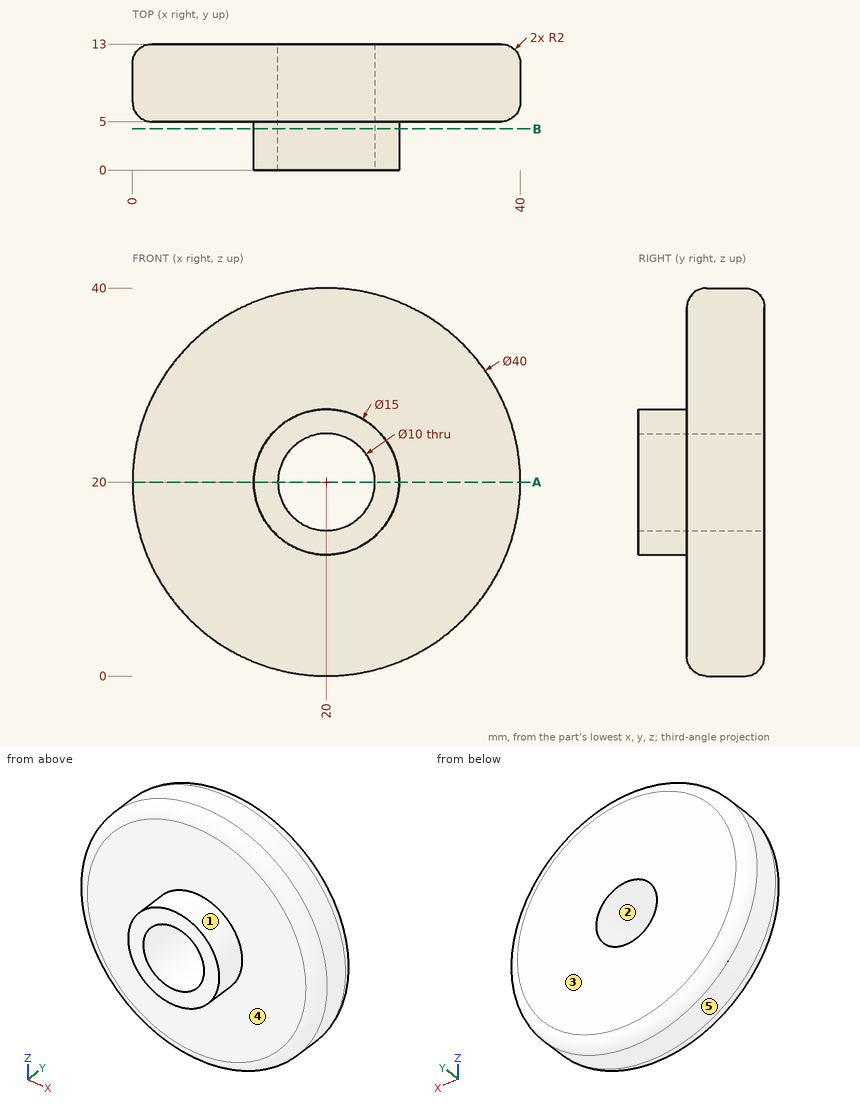
Study the drawing (mm; zero at the part's minimum x, y, z) and answer. A direction names the side the tool comes from. Give positions to 0.01 mm unless a question says otherwise; leave off trailing zeros. Loops run counter-clockwise (first coordinate to the right, second up) from the corner with the lowest first, then second, coordinate; pieces in that order, holes last. Notation, with made-up numbers: (22, 13.25) - (80, 13.25) arc R28 cw to (80, 35.25) - close; hole circle Ø11 at (4, 69.25). An arc over 180 degrees is marked (long way). One line per question, with ' | ' between items.
(1) The part is cut by section A-A (z = 20). Write down the section's boundary in (x, y).
Recorded:
outline: (0, 7) arc R2 ccw to (2, 5) - (12.5, 5) - (12.5, 0) - (15, 0) - (15, 13) - (2, 13) arc R2 ccw to (0, 11) - close; (25, 0) - (27.5, 0) - (27.5, 5) - (38, 5) arc R2 ccw to (40, 7) - (40, 11) arc R2 ccw to (38, 13) - (25, 13) - close
(2) Each of these flat-tipped pins is pushed along its axis until it touches: pin 1 Ø1 at (y, z) = (7.5, 16) entering from +X; pin 2 Ø5 at (y, z) = (9.5, 28) entering from -X; pin 3 Ø6 at (x, y) = (13.5, 8.5) entering from +Z; pin 4 Ø13 at (x, z) = (20, 20) entering from -Y. Where does it stop, or does it pass through?
Recorded:
pin 1: stops at x = 39.69 | pin 2: stops at x = 0.77 | pin 3: stops at z = 39.69 | pin 4: stops at y = 0
(3) The part is cut by section B-B (y = 4.25). Write down the section's boundary in (x, z).
Recorded:
outline: circle Ø15 at (20, 20); hole circle Ø10 at (20, 20)
(4) Straight lines are drawn through the part: probe 1 along Z at (x, y) = (20, 7.5); probe 2 along Z at (x, y) = (20, 4.5); probe 3 along Y at (x, z) = (36, 11.5). For each, find the intervals that lie inside material, in ascending order.
Recorded:
probe 1: z = 0 to 15, 25 to 40 | probe 2: z = 12.5 to 15, 25 to 27.5 | probe 3: y = 5 to 13
(5) The mould has two halves that part along Z. Classify the marked faces 1, 2 and 3: +Z half, -Z half, draft (parallel to the pull), parting line (faces both ways), or undercut.
Recorded:
face 1: parting line | face 2: undercut | face 3: draft
(6) A tool of negligible diameter and unlimited length cuts with its end or side. For the marked faces 4 and 5, from which of +Z, -Z, +X, -X, +Y, -Y can it reach the whole face along a straight path? Write none if from no direction.
Recorded:
face 4: -Y | face 5: +Y, -Y
